Part model, mm, in its own coordinate system. A direction names the side the tool comes from. Round coordinates to 2 decimals unless told otherwise and drop trailing zeros. Loops run counter-clockwise (first coordinate to the right, second up) from the corner with the lowest first, then second, coordinate; pieces in that order, holes last. Notation, with made-up numbers: (12.25, 86.25) -> (31.25, 86.25) arc R10 cw to (31.25, 96.25) -> close; hole circle Ø1 at (52, 24). An arc over 180 degrees is marked (long way). Use a Markdown table: item, result. Add a question column.
Item 1: Cut at D-D, the plane x = -44. List the corners of the cut face in (y, z), plus the area to 3 significant figures.
Item 2: Flat gauge pins, fed straight in: pin 1 (0.6 mm diameter, centred on x = -50.5, z = 26.5, fed in from -Y); pin 2 (1.7 mm diameter, centred on x = -46, y = 3, fed in from +Z); pin 3 (2 mm diameter, centred on y = 31.5, z = 40, fed in from -X). Where does each tip first touch, or does it go through?
Item 3: Cut at C-C, the plane y = 56.6. List the corners of the cut face in (x, z), plus the area to 3 significant figures.
Item 4: Cut at A-A, the plane y = 19.5. List the corners of the cut face in (x, z).
Item 5: Two-plate mould, pull along X, no slides. Class faces 6 (the face through (-42.82, 9.89, 23.85)), 7 (the face through (-48, 12.35, 24)), 8 (the face through (-48.34, 2.94, 23.92)): pulls with the +X half, pulls with the -X half, needs draft (parallel to the pull), parting line crosses it, or undercut.
Item 6: Cut at B-B, the plane z = 24. List the corners of the cut face in (x, y).
Item 7: Which spindle directions (+Z, -Z, +X, -X, +Y, -Y) get a long thin tool onto all of the face, cutting with end or side? Do faces 1 (the face through (-32.69, 32, 38)), 2 (the face through (-48, 52.65, 24)), 3 (the face through (-45, 4, 21.889)), 4 (the face through (-45, 61, 21.889)), 5 (the face through (-48, 56, 26.639)). Say none if no direction does.
Item 8: Probe line 1 (Y direction, x = -53, z = 24.5); line 2 (Z direction, x = -48, y = 7.5); line 3 (X direction, y = 42, z = 30.5). List the from-to ranges inside material, lowest first. Write a range as [from, to].
```python
from build123d import *

# Parameters (mm, degrees)
EXTRUDE_1_DEPTH     = 65
SKETCH_2_W          = 5.5
SKETCH_2_H          = 6.55
EXTRUDE_2_DEPTH     = 20
SKETCH_3_R          = 2.2
CUT_EXTRUDE_1_DEPTH = 20
SKETCH_4_W          = 5.5
SKETCH_4_H          = 6.55
EXTRUDE_3_DEPTH     = 2
RIB_7_REACH         = 67.469
SKETCH_5_WALL_W     = 155.689894758
SKETCH_5_WALL_H     = 4
RIB_8_REACH         = 76.607
SKETCH_6_WALL_W     = 173.96567711
SKETCH_6_WALL_H     = 4


with BuildPart() as part:
    # 草图1 → 凸台-拉伸1 (new body)
    with BuildSketch(Plane(origin=(0, 0, 0), x_dir=(1, 0, 0), z_dir=(0, 1, 0))):
        Polygon((-30.289732276, -35.038566896), (-24.089732276, -35.038566896), (-21.689732276, -37.538566896), (-21.689732276, -39.338566896), (-24.089732276, -39.338566896), (-24.089732276, -41.138566896), (-17.189732276, -41.138566896), (-17.189732276, -21.138566896), (-37.189732276, -21.138566896), (-37.189732276, -41.138566896), (-30.289732276, -41.138566896), (-30.289732276, -39.338566896), (-32.689732276, -39.338566896), (-32.689732276, -37.538566896), align=None)
    extrude(amount=EXTRUDE_1_DEPTH)

    # 草图2 → 凸台-拉伸2 (add)
    with BuildSketch(Plane.ZY.offset(37.189732276)):
        with Locations((23.888566896, 9.075)):
            Rectangle(SKETCH_2_W, SKETCH_2_H)
        with Locations((23.888566896, 55.925)):
            Rectangle(SKETCH_2_W, SKETCH_2_H)
    extrude(amount=EXTRUDE_2_DEPTH)

    # 草图3 → 切除-拉伸1 (cut)
    with BuildSketch(Plane(origin=(0, 0, 21.138566896), x_dir=(-1, 0, 0), z_dir=(0, 0, -1))):
        with Locations((54.339732276, 56.6)):
            Circle(SKETCH_3_R)
        with Locations((44.439732276, 56.6)):
            Circle(SKETCH_3_R)
        with Locations((44.439732276, 8.4)):
            Circle(SKETCH_3_R)
        with Locations((54.339732276, 8.4)):
            Circle(SKETCH_3_R)
    extrude(amount=-CUT_EXTRUDE_1_DEPTH, mode=Mode.SUBTRACT)

    # 草图4 → 凸台-拉伸3 (add)
    with BuildSketch(Plane.ZY.offset(57.189732276)):
        with Locations((23.888566896, 55.925)):
            Rectangle(SKETCH_4_W, SKETCH_4_H)
        with Locations((23.888566896, 9.075)):
            Rectangle(SKETCH_4_W, SKETCH_4_H)
    extrude(amount=EXTRUDE_3_DEPTH)

    # 草图5 wall → 筋7 (add, up to next)
    with BuildSketch(Plane(origin=(-48.189732276, 62.1, 23.888566896), x_dir=(0.966960573226, 0.254925969305, 0), z_dir=(0.254925969305, -0.966960573226, 0)), mode=Mode.PRIVATE) as rib_7_sk1:
        Rectangle(SKETCH_5_WALL_W, SKETCH_5_WALL_H)
    rib_7_tool1 = extrude(rib_7_sk1.sketch, amount=RIB_7_REACH, mode=Mode.PRIVATE) - part.part
    add(rib_7_tool1.solids().sort_by_distance((-48.189732276, 62.1, 23.888566896))[0])

    # 草图6 wall → 筋8 (add, up to next)
    with BuildSketch(Plane(origin=(-48.189732276, 2.9, 23.888566896), x_dir=(0.966960573226, -0.254925969305, 0), z_dir=(-0.254925969305, -0.966960573226, 0)), mode=Mode.PRIVATE) as rib_8_sk1:
        Rectangle(SKETCH_6_WALL_W, SKETCH_6_WALL_H)
    rib_8_tool1 = extrude(rib_8_sk1.sketch, amount=-RIB_8_REACH, mode=Mode.PRIVATE) - part.part
    add(rib_8_tool1.solids().sort_by_distance((-48.189732276, 2.9, 23.888566896))[0])


solid = part.part
```
A:
| question | item | result |
|---|---|---|
| 1 | outline | (1.8, 21.89) -> (5.8, 21.89) -> (5.8, 21.14) -> (6.24, 21.14) -> (6.24, 26.64) -> (5.8, 26.64) -> (5.8, 25.89) -> (1.8, 25.89) -> close; (10.56, 21.14) -> (12.35, 21.14) -> (12.35, 26.64) -> (10.56, 26.64) -> close; (52.65, 21.14) -> (54.44, 21.14) -> (54.44, 26.64) -> (52.65, 26.64) -> close; (58.76, 21.14) -> (59.2, 21.14) -> (59.2, 21.89) -> (63.2, 21.89) -> (63.2, 25.89) -> (59.2, 25.89) -> (59.2, 26.64) -> (58.76, 26.64) -> close |
| 1 | area | 56.7 mm^2 |
| 2 | pin 1 | stops at y = 5.8 |
| 2 | pin 2 | stops at z = 25.89 |
| 2 | pin 3 | stops at x = -37.19 |
| 3 | outline | (-59.19, 21.14) -> (-56.54, 21.14) -> (-56.54, 26.64) -> (-59.19, 26.64) -> close; (-52.14, 21.14) -> (-46.64, 21.14) -> (-46.64, 26.64) -> (-52.14, 26.64) -> close; (-42.24, 21.14) -> (-17.19, 21.14) -> (-17.19, 41.14) -> (-24.09, 41.14) -> (-24.09, 39.34) -> (-21.69, 39.34) -> (-21.69, 37.54) -> (-24.09, 35.04) -> (-30.29, 35.04) -> (-32.69, 37.54) -> (-32.69, 39.34) -> (-30.29, 39.34) -> (-30.29, 41.14) -> (-37.19, 41.14) -> (-37.19, 26.64) -> (-42.24, 26.64) -> close |
| 3 | area | 420 mm^2 |
| 4 | outline | (-37.19, 21.14) -> (-17.19, 21.14) -> (-17.19, 41.14) -> (-24.09, 41.14) -> (-24.09, 39.34) -> (-21.69, 39.34) -> (-21.69, 37.54) -> (-24.09, 35.04) -> (-30.29, 35.04) -> (-32.69, 37.54) -> (-32.69, 39.34) -> (-30.29, 39.34) -> (-30.29, 41.14) -> (-37.19, 41.14) -> close |
| 5 | face 6 | undercut |
| 5 | face 7 | needs draft |
| 5 | face 8 | pulls with the -X half |
| 6 | outline | (-59.19, 5.8) -> (-37.19, 0) -> (-17.19, 0) -> (-17.19, 65) -> (-37.19, 65) -> (-59.19, 59.2) -> (-59.19, 52.65) -> (-37.19, 52.65) -> (-37.19, 12.35) -> (-59.19, 12.35) -> close; hole circle Ø4.4 at (-54.34, 8.4); hole circle Ø4.4 at (-54.34, 56.6); hole circle Ø4.4 at (-44.44, 8.4); hole circle Ø4.4 at (-44.44, 56.6) |
| 7 | face 1 | +Y, -Y |
| 7 | face 2 | +Z, -Z, -X |
| 7 | face 3 | -Z, -X, -Y |
| 7 | face 4 | -Z, -X, +Y |
| 7 | face 5 | +Z, -X, +Y, -Y |
| 8 | line 1 | y = [4.17, 6.65], [10.15, 12.35], [52.65, 54.85], [58.35, 60.83] |
| 8 | line 2 | z = [21.14, 26.64] |
| 8 | line 3 | x = [-37.19, -17.19] |
